Autodesk Inventor part; units mm, degrees
ref_plane "YZ Plane" through (0, 0, 0) normal (1, 0, 0) x (0, 1, 0)
ref_plane "XZ Plane" through (0, 0, 0) normal (0, 1, 0) x (-1, 0, 0)
ref_plane "XY Plane" through (0, 0, 0) normal (0, 0, 1) x (1, 0, 0)
sketch "Sketch1" plane through (0, 0, 0) normal (0, 1, 0) x (-1, 0, 0)
  line L0 (13.8415, 5.1768) -> (-89.2585, 5.1768)
  line L1 (-89.2585, 5.1768) -> (-89.2585, -12.8232)
  line L2 (-89.2585, -12.8232) -> (-79.2585, -12.8232)
  line L3 (-79.2585, -12.8232) -> (-79.2585, -4.5732)
  line L4 (-79.2585, -4.5732) -> (-0.8085, -4.5732)
  line L5 (-0.8085, -4.5732) -> (-0.8085, -11.3232)
  line L6 (-0.8085, -11.3232) -> (13.8415, -11.3232)
  line L7 (13.8415, -11.3232) -> (13.8415, 5.1768)
  circle A0 centre (2.4165, -8.8982) radius 1.325
  circle A1 centre (-83.9335, -9.1482) radius 1.325
  line L8 (13.8415, 5.1768) -> (-89.2585, 5.1768)
  line L9 (-89.2585, 5.1768) -> (-89.2585, 6.1768)
  line L10 (-89.2585, 6.1768) -> (13.8415, 6.1768)
  line L11 (13.8415, 6.1768) -> (13.8415, 5.1768)
  point P0 (0, 0)
  dimension "d0" = 2.65
  dimension "d1" = 2.65
  dimension "d2" = 103.1
  dimension "d3" = 14.65
  dimension "d4" = 10
  dimension "d5" = 18
  dimension "d6" = 16.5
  dimension "d7" = 14.075
  dimension "d8" = 11.425
  dimension "d9" = 9.75
  dimension "d10" = 14.325
  dimension "d11" = 5.325
  dimension "d14" = 1
extrude "Extrusion1" add sketch "Sketch1" along normal blind 1
extrude "Extrusion2" add sketch "Sketch1" against normal blind 7.6 contours L0 L9 L10 L11
sketch "Sketch3" plane through (89.2585, 0, 5.1768) normal (0, 0, -1) x (-1, 0, 0)
  line L0 (103.1, -7.6) -> (0, -7.6)
  line L1 (103.1, -7.6) -> (103.1, 1)
  line L2 (0, -7.6) -> (103.1, -7.6)
  line L3 (103.1, -7.6) -> (103.1, -6.6)
  line L4 (103.1, -6.6) -> (0, -6.6)
  line L5 (0, -6.6) -> (0, -7.6)
  point P0 (89.2585, 0)
  dimension "d17" = 1
extrude "Extrusion3" add sketch "Sketch3" along normal blind 19
properties part number "CO-1-01-jetsonMount"
Geometry: final body of the model. Coordinates: model frame, mm. A direction names the side the tool comes from. Round coordinates to 2 decimals unless told otherwise and drop trailing zeros. Loops run counter-clockwise (first coordinate to the right, second up) from the corner with the lowest first, then second, coordinate; pieces in that order, holes last. Notation, with made-up numbers: (-4.5, 16) -> (15.5, 16) arc R22 cw to (15.5, 35) -> close; hole circle Ø7 at (15, -3.5). An arc over 180 degrees is marked (long way). Use one line per item in the form item = value. Start each with the question number.
1) First-contact query: P1, Ø0.5, axis at x = 47.5, y = 0.5, coming from the -Z side; P2, Ø3.5, axis at x = 37.5, y = -2.5, coming from the -Z side; P3, Ø1, axis at y = -2, z = -4, coming from the +X side; P4, Ø1.5, axis at x = 53.5, z = -10, coming from the +Y side. Flat tips, straight axial feed; report the tip coordinate or a pass-through.
2) Section A-A on z = -1.75. Output: boundary loops of the cut face in (x, y), then the cut area to 3 significant figures.
3) Draft query along Y for faces 4 (the flat face through (37, -7.6, -4)), 5 (the flat face through (38, -3, 6.177)), 6 (the flat face through (38, 0, 0)). Return one class per face: released by +Y, released by -Y, zero draft, split by the parting line, or undercut.
4) Section B-B on x = 39.5. Output: boundary loops of the cut face in (y, z).
5) Access query for faces 1 (the cylindrical face through (83.322, 0.493, -7.973)), 2 (the flat face through (-13.842, -7, -2)), 3 (the flat face through (37, -3, 5.177)). Directions: +Z, -Z, +X, -X, +Y, -Y. A direction counts if a zero-diameter tool reaches every point of the face in a straight line with its end or side. Return the directions, or none.
6) Section C-C on y = -2.5. Output: boundary loops of the cut face in (x, z), then the cut area to 3 significant figures.
7) Line query: L1, parallel to Y at x = 21, z = -3.5; L2, parallel to Y at x = 19.5, z = -9; L3, parallel to Z at x = 54, y = -2.25. Output: solid intervals per line, ascending.
Response:
q1.P1 = -4.57
q1.P2 = 5.18
q1.P3 = through
q1.P4 = -6.6
q2.outline = (-13.84, -7.6) -> (89.26, -7.6) -> (89.26, -6.6) -> (-13.84, -6.6) -> close; (-13.84, 0) -> (89.26, 0) -> (89.26, 1) -> (-13.84, 1) -> close
q2.area = 206 mm^2
q3.face_4 = released by -Y
q3.face_5 = zero draft
q3.face_6 = undercut
q4.outline = (-7.6, -13.82) -> (-6.6, -13.82) -> (-6.6, 5.18) -> (0, 5.18) -> (0, -4.57) -> (1, -4.57) -> (1, 6.18) -> (-7.6, 6.18) -> close
q5.face_1 = +Y
q5.face_2 = +Z, -Z, -X, +Y, -Y
q5.face_3 = -Z, +X, -X
q6.outline = (-13.84, 5.18) -> (89.26, 5.18) -> (89.26, 6.18) -> (-13.84, 6.18) -> close
q6.area = 103 mm^2
q7.L1 = -7.6 to -6.6, 0 to 1
q7.L2 = -7.6 to -6.6
q7.L3 = 5.18 to 6.18
